Study the drawing (mm; zero at the part's minimum x, y, z) and answer. A direction names the side the tool comes from. Coordinates: 2 decimals unless noted, no trailing zeros. Loops run counter-clockwise (first coordinate to the right, second up) from the corner with the lowest first, then second, coordinate; pieces in that order, holes last. Notation, with made-up numbers: (79.5, 64.25) - (117.5, 64.25) arc R23 cw to (117.5, 73.25) - close; hole circle Ø3 at (-11.75, 78). An arc over 180 degrees is marked (long way). Use CSV: the item, a comma, the result in double quotes.
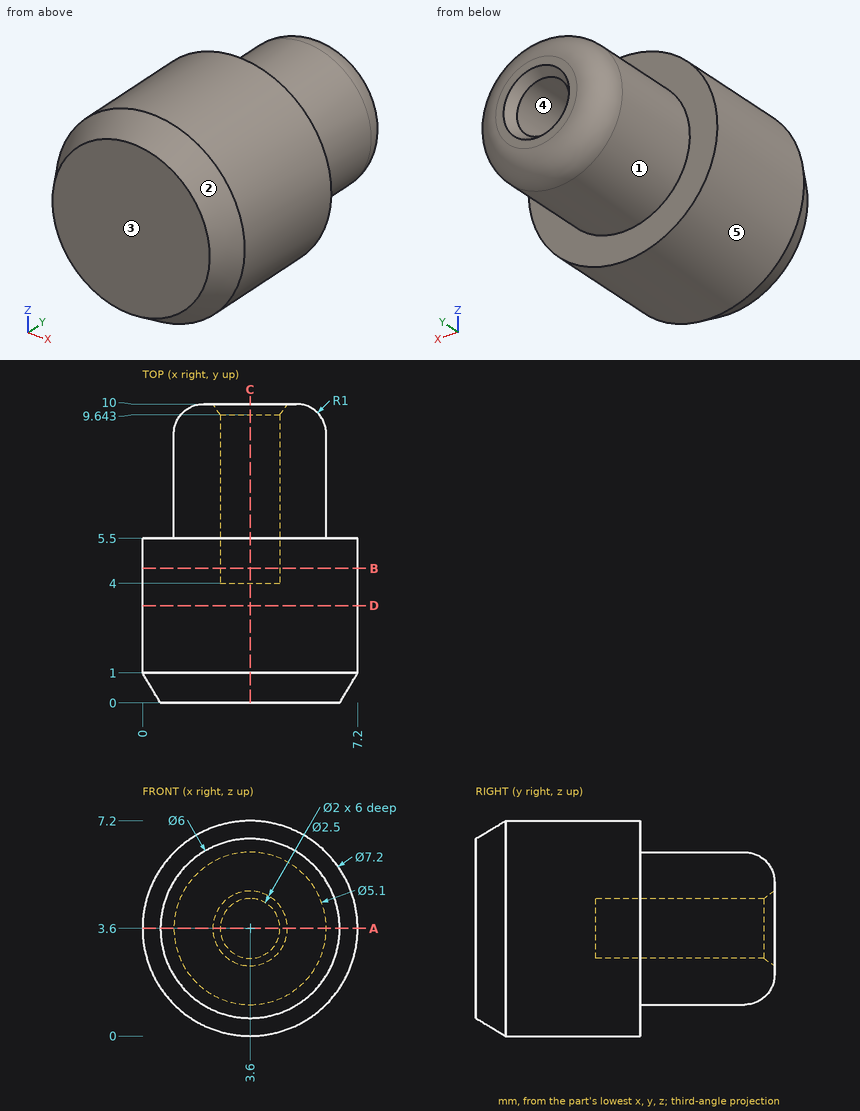
Q1. Given P1, Ø1, axis at x = 3, z = 3, coming from the +Y side, flat-ended and moving along its own axis, determine where the tip first touches the part or whether it passes through.
Reported:
P1,"stops at y = 10"
Q2. The part is cut by section D-D on y = 3.25. Determine the outline of the cut face in (x, z), and give its area (3 significant figures).
Reported:
outline,"circle Ø7.2 at (3.6, 3.6)"
area,"40.7 mm²"
Q3. For a pull along Z with two mould halves and no side action, classify the marked faces 3, 4 and 5 as +Z half, -Z half, draft (parallel to the pull), parting line (faces both ways), or undercut.
Reported:
face 3,"draft"
face 4,"undercut"
face 5,"parting line"
Q4. A tool of negligible diameter and unlimited length cuts with its end or side. For the marked faces 1 and 2, from which of +Z, -Z, +X, -X, +Y, -Y can it reach the whole face along a straight path? Write none if from no direction.
Reported:
face 1,"+Y"
face 2,"-Y"
Q5. The part is cut by section A-A on z = 3.6. Determine the outline of the cut face in (x, y), and give its area (3 significant figures).
Reported:
outline,"(0, 1) - (0.6, 0) - (6.6, 0) - (7.2, 1) - (7.2, 5.5) - (6.15, 5.5) - (6.15, 9) arc R1 ccw to (5.15, 10) - (4.85, 10) - (4.6, 9.64) - (4.6, 4) - (2.6, 4) - (2.6, 9.64) - (2.35, 10) - (2.05, 10) arc R1 ccw to (1.05, 9) - (1.05, 5.5) - (0, 5.5) - close"
area,"49.4 mm²"
Q6. Find the intervals of material crossed by probe 1 along X at (y, z) = (6.3, 3.6); probe 2 along X at (y, z) = (5.4, 3.6); probe 3 along Y at (x, z) = (4, 6.25), in increasing order. Write a range as [from, to].
Reported:
probe 1,"x = [1.05, 2.6], [4.6, 6.15]"
probe 2,"x = [0, 2.6], [4.6, 7.2]"
probe 3,"y = [0, 5.5]"
Q7. The part is cut by section C-C on x = 3.6. Determine the outline of the cut face in (y, z).
Reported:
outline,"(0, 0.6) - (1, 0) - (5.5, 0) - (5.5, 1.05) - (9, 1.05) arc R1 ccw to (10, 2.05) - (10, 2.35) - (9.64, 2.6) - (4, 2.6) - (4, 4.6) - (9.64, 4.6) - (10, 4.85) - (10, 5.15) arc R1 ccw to (9, 6.15) - (5.5, 6.15) - (5.5, 7.2) - (1, 7.2) - (0, 6.6) - close"
Q8. The part is cut by section B-B on y = 4.5. Determine the outline of the cut face in (x, z).
Reported:
outline,"circle Ø7.2 at (3.6, 3.6); hole circle Ø2 at (3.6, 3.6)"
